Input: part model. Units: mm. Frame: model coordinates. A direction names the side the tool comes from. Coordinates: 2 decimals unless noted, no trailing zeros. Write each loop counter-clockwise with the first axis right and the second up, starting at its lowest first coordinate (ties: lowest second). Pieces come first, ordered by that corner, then holes. Notation, with made-up numbers: M 3.25,51.25 L 15.25,51.25 A31 ccw 15.25,88.25 Z; hole C 42,-2 d10. An arc over 180 degrees is marked long. Answer as a JSON object with one key per item and string values. Group by question number.
from build123d import *

# Parameters (mm, degrees)
SKETCH_1_W          = 80
SKETCH_1_H          = 50
EXTRUDE_1_DEPTH     = 1.6
SKETCH_2_W          = 21.2
SKETCH_2_H          = 32.3
EXTRUDE_2_DEPTH     = 13.4
CUT_EXTRUDE_1_DEPTH = 12.7
SKETCH_4_W          = 30
SKETCH_4_H          = 40
EXTRUDE_3_DEPTH     = 10.2
SKETCH_5_W          = 24.26
SKETCH_5_H          = 6.4
CUT_EXTRUDE_2_DEPTH = 63.390704436
CUT_EXTRUDE_3_REACH = 69.068
SKETCH_6_W          = 10
SKETCH_6_H          = 6.4
SKETCH_7_W          = 6.17
SKETCH_7_H          = 3.75
EXTRUDE_4_DEPTH     = 2.4
SKETCH_8_R          = 1.5
CUT_EXTRUDE_4_DEPTH = 1.6
EXTRUDE_5_DEPTH     = 13.8
SKETCH_10_W         = 9
SKETCH_10_H         = 11
EXTRUDE_6_DEPTH     = 3.4
SKETCH_11_R         = 3.15
SKETCH_11_R_2       = 0.85
CUT_EXTRUDE_5_DEPTH = 9.6
FILLET_1_R          = 0.8
SKETCH_12_W         = 30
SKETCH_12_H         = 12.5
EXTRUDE_7_DEPTH     = 2.38
SKETCH_13_W         = 9.62
SKETCH_13_H         = 30
EXTRUDE_8_DEPTH     = 3
SKETCH_14_W         = 9.62
SKETCH_14_H         = 17.5
EXTRUDE_9_DEPTH     = 7
SKETCH_15_R         = 1.5
EXTRUDE_10_DEPTH    = 5.6
SKETCH_16_R         = 0.6
CUT_EXTRUDE_6_DEPTH = 5


with BuildPart() as part:
    # Sketch 1 → Extrude 1 (new body)
    with BuildSketch(Plane(origin=(0, 0, 0), x_dir=(1, 0, 0), z_dir=(0, 1, 0))):
        Rectangle(SKETCH_1_W, SKETCH_1_H)
    extrude(amount=EXTRUDE_1_DEPTH)

    # Sketch 2 → Extrude 2 (add)
    with BuildSketch(Plane(origin=(0, 1.6, 0), x_dir=(1, 0, 0), z_dir=(0, 1, 0))):
        with Locations((30.8, 2.53)):
            Rectangle(SKETCH_2_W, SKETCH_2_H)
    extrude(amount=EXTRUDE_2_DEPTH)

    # Sketch 3 → Cut-Extrude 1 (cut)
    with BuildSketch(Plane(origin=(41.4, 0, 0), x_dir=(0, 0, -1), z_dir=(1, 0, 0))):
        Polygon((0.38, 12.4), (0.38, 5.8), (-2.52, 5.8), (-2.52, 4), (-3.62, 4), (-3.62, 2.6), (-7.62, 2.6), (-7.62, 4), (-8.72, 4), (-8.72, 5.8), (-11.62, 5.8), (-11.62, 12.4), align=None)
        Polygon((12.68, 2.6), (8.68, 2.6), (8.68, 4), (7.58, 4), (7.58, 5.8), (4.68, 5.8), (4.68, 12.4), (16.68, 12.4), (16.68, 5.8), (13.78, 5.8), (13.78, 4), (12.68, 4), align=None)
    extrude(amount=-CUT_EXTRUDE_1_DEPTH, mode=Mode.SUBTRACT)

    # Sketch 4 → Extrude 3 (add)
    with BuildSketch(Plane(origin=(0, 1.6, 0), x_dir=(1, 0, 0), z_dir=(0, 1, 0))):
        with Locations((-4, 0.8)):
            Rectangle(SKETCH_4_W, SKETCH_4_H)
    extrude(amount=EXTRUDE_3_DEPTH)

    # Sketch 5 → Cut-Extrude 2 (cut, through all)
    with BuildSketch(Plane.XY.offset(19.2)):
        with Locations((-4, 4.8)):
            Rectangle(SKETCH_5_W, SKETCH_5_H)
    extrude(amount=-CUT_EXTRUDE_2_DEPTH, mode=Mode.SUBTRACT)

    # Cut-Extrude 3: up to this face of the body (flat: up to its plane)
    cut_extrude_3_end = Plane(part.part.faces().sort_by_distance((11, 6.7, -0.8))[0])
    # Sketch 6 → Cut-Extrude 3 (cut, up to the picked face)
    with BuildSketch(Plane.ZY.offset(19), mode=Mode.PRIVATE) as cut_extrude_3_sk1:
        with Locations((14.2, 4.8)):
            Rectangle(SKETCH_6_W, SKETCH_6_H)
    cut_extrude_3_tool1 = split(extrude(cut_extrude_3_sk1.sketch, amount=-CUT_EXTRUDE_3_REACH, mode=Mode.PRIVATE), bisect_by=cut_extrude_3_end, keep=Keep.BOTH, mode=Mode.PRIVATE)
    add(cut_extrude_3_tool1.solids().sort_by(Axis((-19, 4.8, 14.2), (1, 0, 0)))[0], mode=Mode.SUBTRACT)

    # Sketch 7 → Extrude 4 (add)
    with BuildSketch(Plane(origin=(0, 1.6, 0), x_dir=(1, 0, 0), z_dir=(0, 1, 0))):
        with Locations((17.445, -22.125)):
            Rectangle(SKETCH_7_W, SKETCH_7_H)
        with Locations((28.115, -22.125)):
            Rectangle(SKETCH_7_W, SKETCH_7_H)
    extrude(amount=EXTRUDE_4_DEPTH)

    # Sketch 8 → Cut-Extrude 4 (cut)
    with BuildSketch(Plane(origin=(0, 1.6, 0), x_dir=(1, 0, 0), z_dir=(0, 1, 0))):
        with Locations(Location((16.1, 21.7, 0), (0, 0, 270))):
            Circle(SKETCH_8_R)
        with Locations(Location((15.05, -15.1, 0), (0, 0, 270))):
            Circle(SKETCH_8_R)
        with Locations(Location((-24, -22, 0), (0, 0, 270))):
            Circle(SKETCH_8_R)
        with Locations(Location((-25.7, 21.7, 0), (0, 0, 270))):
            Circle(SKETCH_8_R)
    extrude(amount=-CUT_EXTRUDE_4_DEPTH, mode=Mode.SUBTRACT)

    # Sketch 9 → Extrude 5 (add)
    with BuildSketch(Plane.ZY.offset(41.6)):
        with BuildLine():
            Line((13.495843799, 1.6), (22.495843799, 1.6))
            Line((22.495843799, 1.6), (22.495843799, 7.121383857))
            ThreePointArc((22.495843799, 7.121383857), (17.995843799, 11.621383857), (13.495843799, 7.121383857))
            Line((13.495843799, 7.121383857), (13.495843799, 1.6))
        make_face()
    extrude(amount=-EXTRUDE_5_DEPTH)

    # Sketch 10 → Extrude 6 (add)
    with BuildSketch(Plane.ZY.offset(41.6)):
        with Locations((17.995843799, 7.1)):
            Rectangle(SKETCH_10_W, SKETCH_10_H)
    extrude(amount=-EXTRUDE_6_DEPTH)

    # Sketch 11 → Cut-Extrude 5 (cut)
    with BuildSketch(Plane.ZY.offset(41.6)):
        with Locations((17.995843799, 7.292957317)):
            Circle(SKETCH_11_R)
        with Locations((17.995843799, 7.292957317)):
            Circle(SKETCH_11_R_2, mode=Mode.SUBTRACT)
    extrude(amount=-CUT_EXTRUDE_5_DEPTH, mode=Mode.SUBTRACT)

    # Fillet 1
    fillet_1_edges = [part.edges().sort_by_distance(p)[0] for p in [
        (-41.6, 7.292957317, 17.145843799),
    ]]
    fillet(fillet_1_edges, radius=FILLET_1_R)



with BuildPart() as body_2:
    # Sketch 12 → Extrude 7 (new body)
    with BuildSketch(Plane.ZY.offset(41.6)):
        with Locations((-4.804156201, 7.85)):
            Rectangle(SKETCH_12_W, SKETCH_12_H)
    extrude(amount=-EXTRUDE_7_DEPTH)


with BuildPart() as part_1:
    add(part.part)

    add(body_2.part)  # Extrude 8 merges body 2
    # Sketch 13 → Extrude 8 (add)
    with BuildSketch(Plane(origin=(0, 1.6, 0), x_dir=(1, 0, 0), z_dir=(0, 1, 0))):
        with Locations((-34.41, 4.804156201)):
            Rectangle(SKETCH_13_W, SKETCH_13_H)
    extrude(amount=EXTRUDE_8_DEPTH)

    # Sketch 14 → Extrude 9 (add)
    with BuildSketch(Plane(origin=(0, 4.6, 0), x_dir=(1, 0, 0), z_dir=(0, 1, 0))):
        with Locations((-34.41, 4.804156201)):
            Rectangle(SKETCH_14_W, SKETCH_14_H)
    extrude(amount=EXTRUDE_9_DEPTH)

    # Sketch 15 → Extrude 10 (add)
    # profile 1 of 3: a face of its own
    with BuildSketch(Plane.ZY.offset(41.6)):
        Polygon((-14.009780898, 8.28), (-15.406968549, 10.7), (-18.201343852, 10.7), (-19.598531503, 8.28), (-18.201343852, 5.86), (-15.406968549, 5.86), align=None)
        with Locations((-16.804156201, 8.28)):
            Circle(SKETCH_15_R, mode=Mode.SUBTRACT)
    # profile 2 of 3: a face of its own
    with BuildSketch(Plane.ZY.offset(41.6)):
        Polygon((5.798656148, 5.86), (4.401468497, 8.28), (5.798656148, 10.7), (8.593031451, 10.7), (9.990219102, 8.28), (8.593031451, 5.86), align=None)
        with Locations(Location((7.195843799, 8.28, 0), (0, 0, 180))):
            Circle(SKETCH_15_R, mode=Mode.SUBTRACT)
    # profile 3 of 3: a face of its own
    with BuildSketch(Plane.ZY.offset(41.6)):
        with BuildLine():
            Line((1.695843799, 12.1), (-11.304156201, 12.1))
            ThreePointArc((-11.304156201, 12.1), (-12.507595593, 11.495395794), (-12.740895628, 10.168978172))
            Line((-12.740895628, 10.168978172), (-11.240895628, 5.168978172))
            ThreePointArc((-11.240895628, 5.168978172), (-10.699551995, 4.396560608), (-9.804156201, 4.1))
            Line((-9.804156201, 4.1), (0.195843799, 4.1))
            ThreePointArc((0.195843799, 4.1), (1.091239594, 4.396560608), (1.632583227, 5.168978172))
            Line((1.632583227, 5.168978172), (3.132583227, 10.168978172))
            ThreePointArc((3.132583227, 10.168978172), (2.899283192, 11.495395794), (1.695843799, 12.1))
        make_face()
    extrude(amount=EXTRUDE_10_DEPTH)

    # Sketch 16 → Cut-Extrude 6 (cut)
    with BuildSketch(Plane.ZY.offset(47.2)):
        with Locations((-10.804156201, 9.994214202)):
            Circle(SKETCH_16_R)
        with Locations((-7.804156201, 9.994214202)):
            Circle(SKETCH_16_R)
        with BuildLine():
            ThreePointArc((-4.204156201, 9.994214202), (-4.379892132, 10.41847827), (-4.804156201, 10.594214202))
            Line((-4.804156201, 10.594214202), (-4.804156201, 9.394214202))
            ThreePointArc((-4.804156201, 9.394214202), (-4.379892132, 9.569950133), (-4.204156201, 9.994214202))
        make_face()
        with BuildLine():
            Line((-4.804156201, 9.394214202), (-4.804156201, 10.594214202))
            ThreePointArc((-4.804156201, 10.594214202), (-5.404156201, 9.994214202), (-4.804156201, 9.394214202))
        make_face()
        with Locations((-1.804156201, 9.994214202)):
            Circle(SKETCH_16_R)
        with Locations((1.195843799, 9.994214202)):
            Circle(SKETCH_16_R)
        with Locations((-0.304156201, 7.223993606)):
            Circle(SKETCH_16_R)
        with Locations((-3.304156201, 7.223993606)):
            Circle(SKETCH_16_R)
        with Locations((-6.304156201, 7.223993606)):
            Circle(SKETCH_16_R)
        with Locations((-9.304156201, 7.223993606)):
            Circle(SKETCH_16_R)
    extrude(amount=-CUT_EXTRUDE_6_DEPTH, mode=Mode.SUBTRACT)


solid = part_1.part
Q1. Section A-A, the plane x = -17. Return the cut outline in (y, z), and give its area (3 significant figures).
Q2. Access query for faces 5 (the flat face through (40, 1, 0)), 6 (the flat face through (-40, 14.1, -5)), 7 (the flat face through (-18, 5, 9.2)), 8 (the flat face through (35, 5, -7.58)), 9 (the flat face through (-16.13, 5, -6)). Directions: +Z, -Z, +X, -X, +Y, -Y. A direction counts if a zero-diameter tool reaches every point of the face in a straight line with its end or side. Return the directions, or none.
Q3. Pin query (flat end, axial travel): pin 1 Ø1.9 at (y, z) = (3.5, 21) entering from +X; pin 2 Ø1.9 at (x, z) = (-34, -17.5) entering from +Y; pin 3 Ø1.3 at (x, z) = (-41, 20) entering from -Y; pin 4 Ø1.8 at (x, z) = (-25.7, -21.7) entering from +Y. Return the tip coordinate at first contact, or that it passes through.
Q4. Line query: line 1 (X direction, y = 6.5, z = -9.5); line 2 (X direction, y = 0.5, z = -21.7); line 3 (X direction, y = 2.75, z = -6). Output: solid intervals per line, ascending. Write a range as from..to.
Q5. Draft query along X for faces 1 (the flat face through (-34, 8, -13.554)), 2 (the cylindrical face through (-44.361, 8.346, -18.303)), 3 (the flat face through (20.53, 3, 22)), 4 (the flat face through (41.4, 8, -2)). Return one class per face: released by +X, released by -X, zero draft, split by the parting line, or undercut.
Filled in:
{
 "1": {"outline": "M 0,-25 L 1.6,-25 L 1.6,-20.8 L 11.8,-20.8 L 11.8,19.2 L 8,19.2 L 8,9.2 L 1.6,9.2 L 1.6,25 L 0,25 Z", "area": "424 mm^2"},
 "2": {"face 5": "+Z, -Z, +X, -Y", "face 6": "+Z, -Z, -X, +Y", "face 7": "+Z", "face 8": "+X", "face 9": "+Z, -Z"},
 "3": {"pin 1": "x = 31.2", "pin 2": "y = 4.6", "pin 3": "y = 1.6", "pin 4": "through"},
 "4": {"line 1": "-47.2..-29.6, -19..-16.13, 8.13..11, 20.2..28.7", "line 2": "-40..-27.2, -24.2..14.6, 17.6..40", "line 3": "-41.6..-29.6, -19..-16.13, 8.13..11, 20.2..41.4"},
 "5": {"face 1": "undercut", "face 2": "zero draft", "face 3": "undercut", "face 4": "released by +X"}
}
